Autodesk Fusion 360 part; units mm, degrees
sketch "8x3-Edge_Cuts" plane through (0, 0, 0) normal (0, 0, 1) x (1, 0, 0)
  line L0 (83, -29.5) -> (17, -29.5)
  line L1 (17, -29.5) -> (17, -219.1)
  line L2 (83, -219.1) -> (83, -29.5)
  line L3 (17, -219.1) -> (83, -219.1)
sketch "8x3-User_Drawings" plane through (0, 0, 0) normal (0, 0, 1) x (1, 0, 0)
  circle A0 centre (50.0768, -183.65) radius 9
  circle A1 centre (50.0768, -159.95) radius 9
  circle A2 centre (72.0768, -112.55) radius 9
  circle A3 centre (50.0768, -207.35) radius 9
  circle A4 centre (28.0768, -159.95) radius 9
  circle A5 centre (28.0768, -183.65) radius 9
  circle A6 centre (50.0768, -136.25) radius 9
  circle A7 centre (72.0768, -41.45) radius 9
  circle A8 centre (72.0768, -88.85) radius 9
  circle A9 centre (28.0768, -136.25) radius 9
  circle A10 centre (72.0768, -207.35) radius 9
  circle A11 centre (72.0768, -65.15) radius 9
  circle A12 centre (50.0768, -112.55) radius 9
  circle A13 centre (50.0768, -41.45) radius 9
  circle A14 centre (28.0768, -207.35) radius 9
  circle A15 centre (28.0768, -88.85) radius 9
  circle A16 centre (50.0768, -65.15) radius 9
  circle A17 centre (28.0768, -112.55) radius 9
  circle A18 centre (50.0768, -88.85) radius 9
  circle A19 centre (72.0768, -159.95) radius 9
  circle A20 centre (72.0768, -183.65) radius 9
  circle A21 centre (28.0768, -41.45) radius 9
  circle A22 centre (28.0768, -65.15) radius 9
  circle A23 centre (72.0768, -136.25) radius 9
sketch "8x3-User_Comments" plane through (0, 0, 0) normal (0, 0, 1) x (1, 0, 0)
  circle A0 centre (62.08, -53.72) radius 3
  circle A1 centre (62.58, -195.47) radius 3
  circle A2 centre (61.81, -125.54) radius 3
extrude "Extrude1" add sketch "8x3-Edge_Cuts" along normal blind 2
extrude "Extrude2" cut sketch "8x3-User_Comments" sketch "8x3-User_Drawings" along normal blind 2 of sketch 2
CAD build for the part. Positions are in the model's coordinates, mm. Coordinates: 2 decimals unless noted, no trailing zeros. Order: outer loops, then holes, each group sorted by start corner. A loop starts at its lowest first (then second) coordinate and runs counter-clockwise, first axis right, second up.
(1) Saw through at B-B, the plane z = 1.65. Count the separate pieces of the cut face and the enclosed holes in it, and give its area (3 significant figures).
Solution:
separate pieces: 1
enclosed holes: 27
area: 6,320 mm2
(2) Drill centre lines: L1, parallel to X at y = -41.5, z = 1.1; L2, parallel to X at y = -93, z = 0.7; L3, parallel to X at y = -193, z = 1. Where is each one in solid material? Low to high.
Solution:
L1: x = 17 to 19.08, 37.08 to 41.08, 59.08 to 63.08, 81.08 to 83
L2: x = 17 to 20.09, 36.06 to 42.09, 58.06 to 64.09, 80.06 to 83
L3: x = 17 to 60.88, 64.28 to 83
(3) Saw through at A-A, the plane y = -183.65. Write the cut outline in (x, z).
Solution:
outline: (17, 0) - (19.08, 0) - (19.08, 2) - (17, 2) - close; (37.08, 0) - (41.08, 0) - (41.08, 2) - (37.08, 2) - close; (59.08, 0) - (63.08, 0) - (63.08, 2) - (59.08, 2) - close; (81.08, 0) - (83, 0) - (83, 2) - (81.08, 2) - close
(4) Mould opens along Y. For faces 1 (the face through (65.44, -142.33, 0.99)), 2 (the face through (50, -123, 0)) say: released by +Y, released by -Y, zero draft, split by the parting line, or undercut.
Solution:
face 1: undercut
face 2: zero draft
